Verification items for the finished model (mm, model axes). Face numbers are marked on the shaded views. A direction names the side the tool comes from. Round coordinates to 2 decimals unless told otherwise and drop trailing zeros. Order: outer loops, then holes, each group sorted by start corner. A loop starts at its lowest first (then second) coordinate and runs counter-clockwise, first axis right, second up. Notation, with made-up numbers: (25.25, -36) -> (64.25, -36) arc R12 ccw to (64.25, -30) -> close; hole circle Ø9 at (-32, -18). An arc over 180 degrees is marked (long way). Return JSON: item names as keys, results as strings. Group by question number.
Item 1: Sectioned sample at A-A on z = -10. Record the cut outline in (x, y), plus the area to 3 significant figures.
Item 2: Sectioned sample at D-D on z = 21. Record the cut outline in (x, y), plus the area to 3 significant figures.
Item 3: Depth check by flat-ended pin: pin 1 Ø1 at (y, z) = (27, -13) entering from -X; pin 2 Ø4 at (y, z) = (3.5, -6.5) entering from -X; pin 3 Ø8 at (x, z) = (-2.5, -1.5) entering from +Y. Enter the tip coordinate at first touch or a pass-through.
Item 4: Sectioned sample at C-C on x = 10.5. Record the cut outline in (y, z).
Item 5: Scan lines: probe 1 along Z at (x, y) = (0, 7.75); probe 2 along X at (y, z) = (2.5, 22); probe 3 along Z at (x, y) = (-13, 4). Record each from-to range of solid material in increasing order. Write a range as from..to.
Item 6: Access from +Z, -Z, +X, -X, +Y, -Y to the whole of each face (thin tool, end or side, straight path). Record for the marked faces 1, 2 and 3.
Item 7: Sectioned sample at B-B on y = 43.5. Record the cut outline in (x, z), plus the area to 3 significant figures.
Item 8: Draft check along X on the marked faces 4, 5, 6 and 7. Enter one of: pulls with the +X half, pulls with the -X half, needs draft (parallel to the pull), parting line crosses it, or undercut.
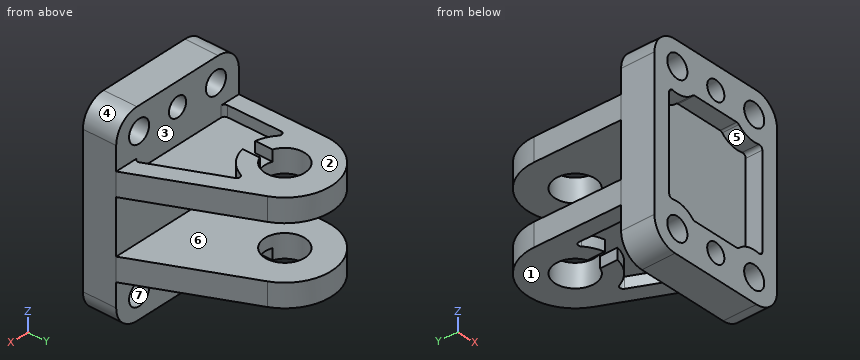
```python
from build123d import *

# Parameters (mm, degrees)
SKETCH1_R               = 3.4
SKETCH1_R_2             = 2.9
BOSS_EXTRUDE1_DEPTH     = 10
CUT_EXTRUDE1_DEPTH      = 5
SKETCH3_R               = 6
BOSS_EXTRUDE2_DEPTH     = 6.95
CUT_EXTRUDE2_DEPTH      = 3.3
SKETCH5_R               = 6
BOSS_EXTRUDE3_DEPTH     = 6.95
CUT_EXTRUDE3_DEPTH      = 3.3
CUT_EXTRUDE4_DEPTH      = 3.3
CUT_EXTRUDE4_DEPTH_BACK = 3.3
CUT_EXTRUDE5_DEPTH      = 3.3
CUT_EXTRUDE5_DEPTH_BACK = 3.3


with BuildPart() as part:
    # Sketch1 → Boss-Extrude1 (new body)
    with BuildSketch(Plane(origin=(0, 0, 0), x_dir=(1, 0, 0), z_dir=(0, 1, 0))):
        with BuildLine():
            Line((-13.75, -29), (13.75, -29))
            ThreePointArc((13.75, -29), (18.699747468, -26.949747468), (20.75, -22))
            Line((20.75, -22), (20.75, 22))
            ThreePointArc((20.75, 22), (18.699747468, 26.949747468), (13.75, 29))
            Line((13.75, 29), (-13.75, 29))
            ThreePointArc((-13.75, 29), (-18.699747468, 26.949747468), (-20.75, 22))
            Line((-20.75, 22), (-20.75, -22))
            ThreePointArc((-20.75, -22), (-18.699747468, -26.949747468), (-13.75, -29))
        make_face()
        with Locations((13, 22)):
            Circle(SKETCH1_R, mode=Mode.SUBTRACT)
        with Locations((13, -22)):
            Circle(SKETCH1_R, mode=Mode.SUBTRACT)
        with Locations((0, 22)):
            Circle(SKETCH1_R_2, mode=Mode.SUBTRACT)
        with Locations((0, -22)):
            Circle(SKETCH1_R_2, mode=Mode.SUBTRACT)
        with Locations((-13, 22)):
            Circle(SKETCH1_R, mode=Mode.SUBTRACT)
        with Locations((-13, -22)):
            Circle(SKETCH1_R, mode=Mode.SUBTRACT)
    extrude(amount=BOSS_EXTRUDE1_DEPTH)

    # Sketch2 → Cut-Extrude1 (cut)
    with BuildSketch(Plane(origin=(0, 0, 0), x_dir=(1, 0, 0), z_dir=(0, 1, 0))):
        with BuildLine():
            Line((-7.121224617, -17), (7.121224617, -17))
            ThreePointArc((7.121224617, -17), (7.499189081, -16.925820104), (7.821078814, -16.714285729))
            ThreePointArc((7.821078814, -16.714285729), (10.936048151, -14.893657568), (14.541666667, -14.762371667))
            ThreePointArc((14.541666667, -14.762371667), (15.37915287, -14.561595372), (15.75, -13.784313784))
            Line((15.75, -13.784313784), (15.75, 13.784313784))
            ThreePointArc((15.75, 13.784313784), (15.379152861, 14.561595378), (14.541666646, 14.762371662))
            ThreePointArc((14.541666646, 14.762371662), (10.936048151, 14.893657568), (7.82107883, 16.714285714))
            ThreePointArc((7.82107883, 16.714285714), (7.49918909, 16.9258201), (7.121224617, 17))
            Line((7.121224617, 17), (-7.121224617, 17))
            ThreePointArc((-7.121224617, 17), (-7.499189081, 16.925820104), (-7.821078814, 16.714285729))
            ThreePointArc((-7.821078814, 16.714285729), (-10.936048151, 14.893657568), (-14.541666667, 14.762371667))
            ThreePointArc((-14.541666667, 14.762371667), (-15.37915287, 14.561595372), (-15.75, 13.784313784))
            Line((-15.75, 13.784313784), (-15.75, -13.784313784))
            ThreePointArc((-15.75, -13.784313784), (-15.379152861, -14.561595378), (-14.541666646, -14.762371662))
            ThreePointArc((-14.541666646, -14.762371662), (-10.936048151, -14.893657568), (-7.82107883, -16.714285714))
            ThreePointArc((-7.82107883, -16.714285714), (-7.49918909, -16.9258201), (-7.121224617, -17))
        make_face()
    extrude(amount=CUT_EXTRUDE1_DEPTH, mode=Mode.SUBTRACT)

    # Sketch3 → Boss-Extrude2 (add)
    with BuildSketch(Plane.XY.offset(15)):
        with BuildLine():
            Line((-20.999349483, 35.865040592), (-20.75, 10))
            Line((-20.75, 10), (20.75, 10))
            Line((20.75, 10), (5.66104691, 41.974771221))
            ThreePointArc((5.66104691, 41.974771221), (-10.127293644, 49.646246168), (-20.999349483, 35.865040592))
        make_face()
        with Locations((-7, 36)):
            Circle(SKETCH3_R, mode=Mode.SUBTRACT)
    extrude(amount=-BOSS_EXTRUDE2_DEPTH)

    # Sketch4 → Cut-Extrude2 (cut)
    with BuildSketch(Plane.XY.offset(15)):
        with BuildLine():
            Line((-15.913359408, 26.969384071), (-15.759315134, 10.990360042))
            ThreePointArc((-15.759315134, 10.990360042), (-15.463051888, 10.289493154), (-14.7593616, 10))
            Line((-14.7593616, 10), (13.643575716, 10))
            ThreePointArc((13.643575716, 10), (14.488196747, 10.464635345), (14.54793621, 11.426769373))
            Line((14.54793621, 11.426769373), (4.956385757, 31.752078197))
            ThreePointArc((4.956385757, 31.752078197), (4.031643534, 32.325101095), (3.131023158, 31.714866422))
            ThreePointArc((3.131023158, 31.714866422), (-4.542840608, 25.277949463), (-14.253955229, 27.73077189))
            ThreePointArc((-14.253955229, 27.73077189), (-15.330435138, 27.887917087), (-15.913359408, 26.969384071))
        make_face()
    extrude(amount=-CUT_EXTRUDE2_DEPTH, mode=Mode.SUBTRACT)

    # Sketch5 → Boss-Extrude3 (add)
    with BuildSketch(Plane.XY.offset(-15)):
        with BuildLine():
            Line((-20.999349483, 35.865040592), (-20.75, 10))
            Line((-20.75, 10), (20.75, 10))
            Line((20.75, 10), (5.66104691, 41.974771221))
            ThreePointArc((5.66104691, 41.974771221), (-10.127293644, 49.646246168), (-20.999349483, 35.865040592))
        make_face()
        with Locations((-7, 36)):
            Circle(SKETCH5_R, mode=Mode.SUBTRACT)
    extrude(amount=BOSS_EXTRUDE3_DEPTH)

    # Sketch6 → Cut-Extrude3 (cut)
    with BuildSketch(Plane.XY.offset(-15)):
        with BuildLine():
            Line((-15.913359408, 26.969384071), (-15.759315134, 10.990360042))
            ThreePointArc((-15.759315134, 10.990360042), (-15.463051888, 10.289493154), (-14.7593616, 10))
            Line((-14.7593616, 10), (13.643575716, 10))
            ThreePointArc((13.643575716, 10), (14.488196747, 10.464635345), (14.54793621, 11.426769373))
            Line((14.54793621, 11.426769373), (4.956385757, 31.752078197))
            ThreePointArc((4.956385757, 31.752078197), (4.031643534, 32.325101095), (3.131023158, 31.714866422))
            ThreePointArc((3.131023158, 31.714866422), (-4.542840608, 25.277949463), (-14.253955229, 27.73077189))
            ThreePointArc((-14.253955229, 27.73077189), (-15.330435138, 27.887917087), (-15.913359408, 26.969384071))
        make_face()
    extrude(amount=CUT_EXTRUDE3_DEPTH, mode=Mode.SUBTRACT)

    # Sketch7 → Cut-Extrude4 (cut, two sides)
    with BuildSketch(Plane.XY.offset(15)) as cut_extrude4_sk:
        with BuildLine():
            Line((-4.85, 23.15), (-4.85, 36))
            Line((-4.85, 36), (-9.15, 36))
            Line((-9.15, 36), (-9.15, 23.15))
            ThreePointArc((-9.15, 23.15), (-7, 21), (-4.85, 23.15))
        make_face()
    extrude(amount=CUT_EXTRUDE4_DEPTH, mode=Mode.SUBTRACT)
    extrude(cut_extrude4_sk.sketch, amount=-CUT_EXTRUDE4_DEPTH_BACK, mode=Mode.SUBTRACT)

    # Sketch8 → Cut-Extrude5 (cut, two sides)
    with BuildSketch(Plane.XY.offset(-15)) as cut_extrude5_sk:
        with BuildLine():
            Line((-4.85, 23.15), (-4.85, 36))
            Line((-4.85, 36), (-9.15, 36))
            Line((-9.15, 36), (-9.15, 23.15))
            ThreePointArc((-9.15, 23.15), (-7, 21), (-4.85, 23.15))
        make_face()
    extrude(amount=CUT_EXTRUDE5_DEPTH, mode=Mode.SUBTRACT)
    extrude(cut_extrude5_sk.sketch, amount=-CUT_EXTRUDE5_DEPTH_BACK, mode=Mode.SUBTRACT)


solid = part.part
```
Recorded:
{
 "1": {"outline": "(-21, 35.87) -> (-20.75, 10) -> (-20.75, 0) -> (-15.75, 0) -> (-15.75, 5) -> (15.75, 5) -> (15.75, 0) -> (20.75, 0) -> (20.75, 10) -> (5.66, 41.97) arc R14 ccw to start; hole circle Ø12 at (-7, 36)", "area": "1,380 mm²"},
 "2": {"outline": "(-20.75, 0) -> (-16.25, 0) -> (-16.25, 10) -> (-20.75, 10) -> close; (-9.75, 0) -> (-2.72, 0) -> (-2.72, 10) -> (-9.75, 10) -> close; (2.72, 0) -> (9.75, 0) -> (9.75, 10) -> (2.72, 10) -> close; (16.25, 0) -> (20.75, 0) -> (20.75, 10) -> (16.25, 10) -> close", "area": "231 mm²"},
 "3": {"pin 1": "x = -20.92", "pin 2": "x = -20.75", "pin 3": "y = 10"},
 "4": {"outline": "(0, -29) -> (10, -29) -> (10, -24.3) -> (0, -24.3) -> close; (0, -19.7) -> (10, -19.7) -> (10, -11.7) -> (20, -11.7) -> (20, -15) -> (31.72, -15) -> (31.72, -8.05) -> (10, -8.05) -> (10, 8.05) -> (31.72, 8.05) -> (31.72, 15) -> (20, 15) -> (20, 11.7) -> (10, 11.7) -> (10, 19.7) -> (0, 19.7) -> (0, 15.04) -> (5, 15.04) -> (5, -15.04) -> (0, -15.04) -> close; (0, 24.3) -> (10, 24.3) -> (10, 29) -> (0, 29) -> close"},
 "5": {"probe 1": "-29..-24.9, -19.1..19.1, 24.9..29", "probe 2": "-20.75..-16.4, -9.6..-2.9, 2.9..9.6, 16.4..20.75", "probe 3": "-29..-25.4, -18.6..-14.6, 14.6..18.6, 25.4..29"},
 "6": {"face 1": "-Z, +X, -X, +Y", "face 2": "+Z, +X, -X, +Y", "face 3": "+Z"},
 "7": {"outline": "(-18.82, -15) -> (4.82, -15) -> (4.82, -8.05) -> (-18.82, -8.05) -> close; (-18.82, 8.05) -> (4.82, 8.05) -> (4.82, 15) -> (-18.82, 15) -> close", "area": "329 mm²"},
 "8": {"face 4": "pulls with the +X half", "face 5": "undercut", "face 6": "needs draft", "face 7": "undercut"}
}
